from build123d import *

# Parameters (mm, degrees)
SKETCH1_R                   = 7.9375
SKETCH1_R_2                 = 11.1125
BOSS_EXTRUDE1_DEPTH         = 12.7
F_8_CLEARANCE_HOLE1_D       = 4.4958
SKETCH5_R                   = 18.415
CUT_EXTRUDE1_DEPTH          = 13.7
SKETCH7_R                   = 9.525
CUT_EXTRUDE2_DEPTH          = 13.7
CUT_EXTRUDE3_DEPTH          = 13.7
BOSS_EXTRUDE2_DEPTH         = 12.7
CUT_EXTRUDE4_DEPTH          = 13.7
SKETCH11_W                  = 12.7
SKETCH11_H                  = 178.054
CUT_EXTRUDE5_DEPTH          = 3.175
BOSS_EXTRUDE3_DEPTH         = 6.35
CUT_EXTRUDE6_DEPTH          = 13.7
F_3_8_CLEARANCE_HOLE1_D     = 10.0838
F_3_8_CLEARANCE_HOLE1_DEPTH = 12.7
F_3_8_CLEARANCE_HOLE1_TIP   = 3.029479155
FILLET1_R                   = 12.7
SKETCH16_W                  = 6.35
SKETCH16_H                  = 25.4
BOSS_EXTRUDE4_DEPTH         = 6.35


with BuildPart() as part:
    # Sketch1 → Boss-Extrude1 (new body)
    with BuildSketch(Plane(origin=(0, 0, 0), x_dir=(0, 0, -1), z_dir=(1, 0, 0))):
        with BuildLine():
            Line((93.345, 0), (55.245, 50.8))
            Line((55.245, 50.8), (-160.655, 50.8))
            ThreePointArc((-160.655, 50.8), (-211.455, 0), (-160.655, -50.8))
            Line((-160.655, -50.8), (55.245, -50.8))
            Line((55.245, -50.8), (93.345, 0))
        make_face()
        with Locations((-88.9, 0)):
            Circle(SKETCH1_R, mode=Mode.SUBTRACT)
        with Locations((-38.1, 0)):
            Circle(SKETCH1_R, mode=Mode.SUBTRACT)
        with Locations((-160.655, 0)):
            Circle(SKETCH1_R_2, mode=Mode.SUBTRACT)
        Circle(SKETCH1_R, mode=Mode.SUBTRACT)
    extrude(amount=BOSS_EXTRUDE1_DEPTH)

    # #8 Clearance Hole1 (through all)
    with Locations(Plane.ZY):
        with Locations((-17.691104559, 17.691104559), (17.691104559, 17.691104559), (17.691104559, -17.691104559), (-17.691104559, -17.691104559)):
            Hole(F_8_CLEARANCE_HOLE1_D / 2)

    # Sketch5 → Cut-Extrude1 (cut, through all)
    with BuildSketch(Plane.ZY):
        Circle(SKETCH5_R)
    extrude(amount=-CUT_EXTRUDE1_DEPTH, mode=Mode.SUBTRACT)

    # Sketch7 → Cut-Extrude2 (cut, through all)
    with BuildSketch(Plane.ZY):
        with Locations((-55.245, 0)):
            Circle(SKETCH7_R)
    extrude(amount=-CUT_EXTRUDE2_DEPTH, mode=Mode.SUBTRACT)

    # Sketch8 → Cut-Extrude3 (cut, through all)
    with BuildSketch(Plane(origin=(12.7, 0, 0), x_dir=(0, 0, -1), z_dir=(1, 0, 0))):
        Polygon((-160.655, 50.8), (-211.455, 25.4), (-211.455, -25.4), (-160.655, -50.8), (-233.239745749, -50.8), (-233.239745749, 50.8), align=None)
    extrude(amount=-CUT_EXTRUDE3_DEPTH, mode=Mode.SUBTRACT)

    # Sketch9 → Boss-Extrude2 (add)
    with BuildSketch(Plane(origin=(12.7, 0, 0), x_dir=(0, 0, -1), z_dir=(1, 0, 0))):
        Polygon((-160.655, 50.8), (-211.455, 25.4), (-211.455, 0), (-211.455, -25.4), (-160.655, -50.8), (-160.655, -40.64), (-202.749323348, 0), (-160.655, 40.64), align=None)
    extrude(amount=-BOSS_EXTRUDE2_DEPTH)

    # Sketch10 → Cut-Extrude4 (cut, through all)
    with BuildSketch(Plane.ZY):
        Polygon((-79.0575, -19.05), (-79.0575, 19.05), (-93.345, 0), align=None)
    extrude(amount=-CUT_EXTRUDE4_DEPTH, mode=Mode.SUBTRACT)

    # Sketch11 → Cut-Extrude5 (cut)
    with BuildSketch(Plane(origin=(0, 50.8, 0), x_dir=(1, 0, 0), z_dir=(0, 1, 0))):
        with Locations((6.35, -52.705)):
            Rectangle(SKETCH11_W, SKETCH11_H)
    cut_extrude5 = extrude(amount=-CUT_EXTRUDE5_DEPTH, mode=Mode.SUBTRACT)

    # Mirror1: Cut-Extrude5 across plane
    add(cut_extrude5.mirror(Plane.ZX), mode=Mode.SUBTRACT)

    # Sketch13 → Cut-Extrude6 (cut, through all)
    with BuildSketch(Plane(origin=(12.7, 0, 0), x_dir=(0, 0, -1), z_dir=(1, 0, 0))):
        Polygon((-161.254612663, -53.34), (-139.192, -53.34), (-139.192, -50.165), (33.782, -50.165), (33.782, -53.34), (56.515, -53.34), (81.5975, -19.896666667), (81.5975, 19.896666667), (56.515, 53.34), (33.782, 53.34), (33.782, 50.165), (-139.192, 50.165), (-139.192, 53.34), (-161.254612663, 53.34), (-213.995, 26.969806331), (-213.995, -26.969806331), align=None)
    extrude(amount=-CUT_EXTRUDE6_DEPTH, mode=Mode.SUBTRACT)


with BuildPart() as body_2:
    # Sketch12 → Boss-Extrude3 (new body)
    with BuildSketch(Plane(origin=(12.7, 0, 0), x_dir=(0, 0, -1), z_dir=(1, 0, 0))):
        with BuildLine():
            ThreePointArc((-211.89681554, -56.397839854), (-236.855, 0), (-211.89681554, 56.397839854))
            Line((-211.89681554, 56.397839854), (-243.205, 43.989212666))
            Line((-243.205, 43.989212666), (-243.205, -43.989212666))
            Line((-243.205, -43.989212666), (-211.89681554, -56.397839854))
        make_face()
        with BuildLine():
            Line((-217.805, 29.324515829), (-162.154031657, 57.15))
            Line((-162.154031657, 57.15), (-166.916531657, 66.675))
            Line((-166.916531657, 66.675), (-185.966531657, 66.675))
            Line((-185.966531657, 66.675), (-211.89681554, 56.397839854))
            ThreePointArc((-211.89681554, 56.397839854), (-236.855, 0), (-211.89681554, -56.397839854))
            Line((-211.89681554, -56.397839854), (-185.966531657, -66.675))
            Line((-185.966531657, -66.675), (-166.916531657, -66.675))
            Line((-166.916531657, -66.675), (-162.154031657, -57.15))
            Line((-162.154031657, -57.15), (-217.805, -29.324515829))
            Line((-217.805, -29.324515829), (-217.805, 29.324515829))
        make_face()
    extrude(amount=-BOSS_EXTRUDE3_DEPTH)

    # 3/8 Clearance Hole1
    with Locations(Plane(origin=(12.7, 0, 0), x_dir=(0, 0, -1), z_dir=(1, 0, 0))):
        with Locations((-230.505, 0), (-230.505, 33.690140829), (-202.106936686, 47.889172486), (-230.505, -33.690140829), (-202.106936686, -47.889172486)):
            Hole(F_3_8_CLEARANCE_HOLE1_D / 2, depth=F_3_8_CLEARANCE_HOLE1_DEPTH)
            with Locations((0, 0, -(F_3_8_CLEARANCE_HOLE1_DEPTH + F_3_8_CLEARANCE_HOLE1_TIP / 2))):  # 118° drill point
                Cone(0, F_3_8_CLEARANCE_HOLE1_D / 2, F_3_8_CLEARANCE_HOLE1_TIP, mode=Mode.SUBTRACT)

    # Fillet1
    fillet1_edges = [body_2.edges().sort_by_distance(p)[0] for p in [
        (9.525, -43.989212666, 243.205),
        (9.525, 43.989212666, 243.205),
        (9.525, 66.675, 185.966531657),
        (9.525, 66.675, 166.916531657),
        (9.525, -66.675, 166.916531657),
        (9.525, -66.675, 185.966531657),
    ]]
    fillet(fillet1_edges, radius=FILLET1_R)

    # Sketch16 → Boss-Extrude4 (add)
    with BuildSketch(Plane(origin=(12.7, 0, 0), x_dir=(0, 0, -1), z_dir=(1, 0, 0))):
        with Locations((-214.63, 0)):
            Rectangle(SKETCH16_W, SKETCH16_H)
        Polygon((-178.620290503, -48.916870577), (-175.780484171, -43.237257914), (-198.498934823, -31.878032589), (-201.338741154, -37.557645251), align=None)
        Polygon((-201.338741154, 37.557645251), (-198.498934823, 31.878032589), (-175.780484171, 43.237257914), (-178.620290503, 48.916870577), align=None)
    extrude(amount=-BOSS_EXTRUDE4_DEPTH)


solid = body_2.part
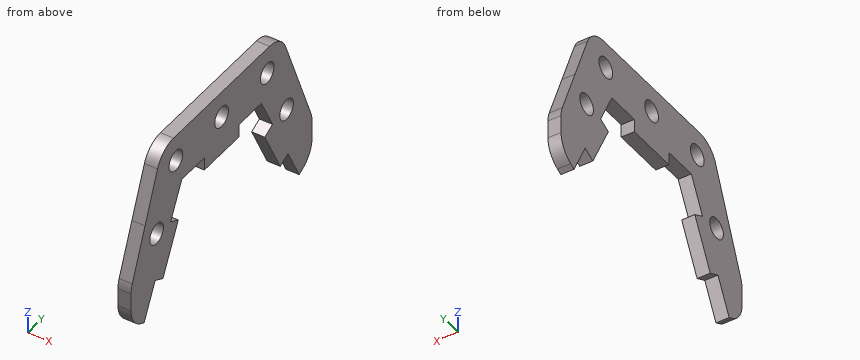
Geometry: final body of the model. Coordinates: model frame, mm. Round coordinates to 2 decimals unless told otherwise and drop trailing zeros. Order: outer loops, then holes, each group sorted by start corner. A loop starts at its lowest first (then second) coordinate and runs counter-clockwise, first axis right, second up.
Q1. Material intervals for probe 1 along Y at (x, z) = (8, 217); probe 2 along Z at (x, y) = (10.25, -34.5) (3 decimals); probe 3 along Y at (x, z) = (11.5, 227), sorted ascending.
Result sheet:
probe 1: y = -54.38 to -29.73, -12.7 to 12.7, 29.73 to 54.38
probe 2: z = 193.255 to 199.81, 207.454 to 225.529, 235.481 to 243.205
probe 3: y = -50.41 to -37.31, -30.07 to -3.62, 3.62 to 30.07, 37.31 to 50.41
Q2. Section A-A, the plane y = 0. Output: boundary loops of the cut face in (x, z) (3 decimals).
Result sheet:
outline: (6.35, 211.455) - (12.7, 211.455) - (12.7, 225.463) - (6.35, 225.463) - close; (6.35, 235.547) - (12.7, 235.547) - (12.7, 243.205) - (6.35, 243.205) - close
Q3. Pin query (flat end, axial travel): pin 1 (1.9 mm diameter, centred on x = 10.5, z = 214, fed in from +Y); pin 2 (1.9 mm diameter, centred on x = 10.5, y = 22.5, fed in from -Z) (3 decimals); pin 3 (6 mm diameter, centred on y = 47.89, z = 202.11, fed in from -X); pin 4 (1.5 mm diameter, centred on x = 9, y = -30, fed in from -Z). Return the tip coordinate at first contact, or that it passes through.
Result sheet:
pin 1: stops at y = 55.94
pin 2: stops at z = 217.805
pin 3: passes through
pin 4: stops at z = 214.95
Q4. Section C-C, the plane x = 8. Give the number of separate pieces and of enclosed holes in the cut face, and give its area (3 significant figures).
Result sheet:
separate pieces: 1
enclosed holes: 5
area: 4,690 mm2
Q5. Section D-D, the plane y = -22.5. Output: boundary loops of the cut face in (x, z) (3 decimals).
Result sheet:
outline: (6.35, 217.805) - (12.7, 217.805) - (12.7, 243.205) - (6.35, 243.205) - close
Q6. Section B-B, the plane z = 190.5. Output: boundary loops of the cut face in (x, y).
Result sheet:
outline: (6.35, -64.88) - (12.7, -64.88) - (12.7, -35.88) - (6.35, -35.88) - close; (6.35, 35.88) - (12.7, 35.88) - (12.7, 64.88) - (6.35, 64.88) - close
